Here's how the part is built. I have some questions about the finished solid (model axes, mm). Give positions to 0.01 mm unless a question says otherwise; leave off trailing zeros. Loops run counter-clockwise (first coordinate to the right, second up) from the corner with the lowest first, then second, coordinate; pieces in that order, holes last. Notation, with made-up numbers: (43.5, 26.5) - (52.5, 26.5) arc R15 cw to (52.5, 55.5) - close; hole circle Ø11 at (17.5, -11). An arc over 180 degrees is marked (long way). Return JSON: item names as keys, results as strings. Group by question number.
(1) I need wall thicknesses on probe 1 along X at (y, z) = (5.65, 171.5); probe 2 along Z at (x, y) = (46, 4.2); probe 3 along Z at (x, y) = (45, 1.7). Which ranges of each line are inside material? Lowest first, please. Write a range as [from, to].
(2) If we section it at A-A (z = 181.5): Please give me the cut outline in (x, y).
(3) For P1, Ø3, axis at x = 11, y = 1.5, coming from the +Z side; P2, Ø1.8, axis at y = 2, z = 282, coming from the -X side, each with a flat end and sliding along its axis, tell me the tip position at first contact or that it passes through.
(4) If we section it at B-B (y = 2.25): State how many separate pieces and enclosed holes the cut face has, then the cut area to 3 significant figures.
```python
from build123d import *

# Parameters (mm, degrees)
SKETCH1_W                 = 60.2
SKETCH1_H                 = 160
BOSS_EXTRUDE1_DEPTH       = 6
BOSS_EXTRUDE2_START       = -6
BOSS_EXTRUDE2_OUTLINE_W   = 140.2
BOSS_EXTRUDE2_OUTLINE_H   = 468.2
BOSS_EXTRUDE2_OUTLINE_W_2 = 60.2
BOSS_EXTRUDE2_OUTLINE_H_2 = 160
BOSS_EXTRUDE2_DEPTH       = 6
SKETCH3_W                 = 5.8
SKETCH3_H                 = 70.8
CUT_EXTRUDE1_DEPTH        = 6
SKETCH4_W                 = 30
SKETCH4_H                 = 6
BOSS_EXTRUDE3_DEPTH       = 6


# Read off the part's stored shape, not the designer's step: Boss-Extrude2
with BuildPart() as part:
    # Sketch1 → Boss-Extrude1 (new body)
    with BuildSketch(Plane(origin=(0, 0, 0), x_dir=(1, 0, 0), z_dir=(0, 1, 0))):
        with Locations((30.1, 80)):
            Rectangle(SKETCH1_W, SKETCH1_H)
        with BuildLine():
            Line((7.85, 152.55), (16.15, 152.55))
            ThreePointArc((16.15, 152.55), (19.6, 149.1), (16.15, 145.65))
            Line((16.15, 145.65), (7.85, 145.65))
            ThreePointArc((7.85, 145.65), (4.4, 149.1), (7.85, 152.55))
        make_face(mode=Mode.SUBTRACT)
        with BuildLine():
            Line((44.05, 145.65), (52.35, 145.65))
            ThreePointArc((52.35, 145.65), (55.8, 149.1), (52.35, 152.55))
            Line((52.35, 152.55), (44.05, 152.55))
            ThreePointArc((44.05, 152.55), (40.6, 149.1), (44.05, 145.65))
        make_face(mode=Mode.SUBTRACT)
        with BuildLine():
            Line((52.35, 7.45), (44.05, 7.45))
            ThreePointArc((44.05, 7.45), (40.6, 10.9), (44.05, 14.35))
            Line((44.05, 14.35), (52.35, 14.35))
            ThreePointArc((52.35, 14.35), (55.8, 10.9), (52.35, 7.45))
        make_face(mode=Mode.SUBTRACT)
        with BuildLine():
            Line((16.15, 14.35), (7.85, 14.35))
            ThreePointArc((7.85, 14.35), (4.4, 10.9), (7.85, 7.45))
            Line((7.85, 7.45), (16.15, 7.45))
            ThreePointArc((16.15, 7.45), (19.6, 10.9), (16.15, 14.35))
        make_face(mode=Mode.SUBTRACT)
    extrude(amount=BOSS_EXTRUDE1_DEPTH)

    # Boss-Extrude2 outline → Boss-Extrude2 (add)
    with BuildSketch(Plane(origin=(0, 6, 0), x_dir=(1, 0, 0), z_dir=(0, 1, 0)).offset(BOSS_EXTRUDE2_START)):
        with Locations((30.1, -45)):
            Rectangle(BOSS_EXTRUDE2_OUTLINE_W, BOSS_EXTRUDE2_OUTLINE_H)
        with Locations((30.1, 80)):
            Rectangle(BOSS_EXTRUDE2_OUTLINE_W_2, BOSS_EXTRUDE2_OUTLINE_H_2, mode=Mode.SUBTRACT)
    extrude(amount=BOSS_EXTRUDE2_DEPTH)

    # Sketch3 → Cut-Extrude1 (cut)
    with BuildSketch(Plane(origin=(0, 6, 0), x_dir=(1, 0, 0), z_dir=(0, 1, 0))):
        with Locations((87.3, 122.8465093)):
            Rectangle(SKETCH3_W, SKETCH3_H)
        with Locations((-27.1, 122.8465093)):
            Rectangle(SKETCH3_W, SKETCH3_H)
        with Locations((-27.1, -27.1534907)):
            Rectangle(SKETCH3_W, SKETCH3_H)
        with Locations((87.3, -27.1534907)):
            Rectangle(SKETCH3_W, SKETCH3_H)
        with Locations((-27.1, -177.1534907)):
            Rectangle(SKETCH3_W, SKETCH3_H)
        with Locations((87.3, -177.1534907)):
            Rectangle(SKETCH3_W, SKETCH3_H)
    extrude(amount=-CUT_EXTRUDE1_DEPTH, mode=Mode.SUBTRACT)

    # Sketch4 → Boss-Extrude3 (add)
    with BuildSketch(Plane(origin=(0, 6, 0), x_dir=(1, 0, 0), z_dir=(0, 1, 0))):
        with Locations((-12, -282.1)):
            Rectangle(SKETCH4_W, SKETCH4_H)
        with Locations((30.1, -282.1)):
            Rectangle(SKETCH4_W, SKETCH4_H)
        with Locations((72.2, -282.1)):
            Rectangle(SKETCH4_W, SKETCH4_H)
    extrude(amount=-BOSS_EXTRUDE3_DEPTH)


solid = part.part
```
Values:
{
 "1": {"probe 1": "[-40, -30], [-24.2, 84.4], [90.2, 100.2]", "probe 2": "[-189.1, -152.55], [-145.65, -14.35], [-7.45, 279.1]", "probe 3": "[-189.1, -152.55], [-145.65, -14.35], [-7.45, 285.1]"},
 "2": {"outline": "(-40, 0) - (-30, 0) - (-30, 6) - (-40, 6) - close; (-24.2, 0) - (84.4, 0) - (84.4, 6) - (-24.2, 6) - close; (90.2, 0) - (100.2, 0) - (100.2, 6) - (90.2, 6) - close"},
 "3": {"P1": "z = 279.1", "P2": "x = -27"},
 "4": {"separate pieces": "1", "enclosed holes": "10", "area": "63,300 mm2"}
}
